```python
from build123d import *

# Parameters (mm, degrees)
F0_W     = 10
F0_H     = 3.175
F0_W_2   = 51.432349664
F0_H_2   = 65
F0_R     = 1.64084
F0_W_3   = 39.0626990616
F0_H_3   = 50
F1_DEPTH = 3.175


# Not quite as in the source:
# - a feature names something its author has since deleted; it is built from what else it names


with BuildPart() as f1:
    # F0 (on Front) → F1 (new body)
    with BuildSketch(Plane.XZ):
        with BuildLine():
            Line((79.2994276966, -35.2024036679), (122.1565705538, -35.2024036679))
            Line((122.1565705538, -35.2024036679), (122.1565705538, 64.7975963321))
            Line((122.1565705538, 64.7975963321), (79.2994276966, 64.7975963321))
            Line((79.2994276966, 64.7975963321), (79.2994276966, 67.9725963321))
            Line((79.2994276966, 67.9725963321), (7.870856268, 67.9725963321))
            Line((7.870856268, 67.9725963321), (7.870856268, 64.7975963321))
            Line((7.870856268, 64.7975963321), (-63.5577151605, 64.7975963321))
            Line((-63.5577151605, 64.7975963321), (-63.5577151605, 67.9725963321))
            Line((-63.5577151605, 67.9725963321), (-134.9862865891, 67.9725963321))
            Line((-134.9862865891, 67.9725963321), (-134.9862865891, 64.7975963321))
            Line((-134.9862865891, 64.7975963321), (-206.4148580177, 64.7975963321))
            Line((-206.4148580177, 64.7975963321), (-206.4148580177, 67.9725963321))
            Line((-206.4148580177, 67.9725963321), (-277.8434294462, 67.9725963321))
            Line((-277.8434294462, 67.9725963321), (-277.8434294462, 64.7975963321))
            Line((-277.8434294462, 64.7975963321), (-277.8434294462, 18.0995963321))
            ThreePointArc((-277.8434294462, 18.0995963321), (-275.5085628548, 17.1324629236), (-274.5414294462, 14.7975963321))
            ThreePointArc((-274.5414294462, 14.7975963321), (-275.5085628548, 12.4627297406), (-277.8434294462, 11.4955963321))
            Line((-277.8434294462, 11.4955963321), (-277.8434294462, -35.2024036679))
            Line((-277.8434294462, -35.2024036679), (-277.8434294462, -38.3774036679))
            Line((-277.8434294462, -38.3774036679), (-206.4148580177, -38.3774036679))
            Line((-206.4148580177, -38.3774036679), (-206.4148580177, -35.2024036679))
            Line((-206.4148580177, -35.2024036679), (-134.9862865891, -35.2024036679))
            Line((-134.9862865891, -35.2024036679), (-134.9862865891, -38.3774036679))
            Line((-134.9862865891, -38.3774036679), (-63.5577151605, -38.3774036679))
            Line((-63.5577151605, -38.3774036679), (-63.5577151605, -35.2024036679))
            Line((-63.5577151605, -35.2024036679), (7.870856268, -35.2024036679))
            Line((7.870856268, -35.2024036679), (7.870856268, -38.3774036679))
            Line((7.870856268, -38.3774036679), (79.2994276966, -38.3774036679))
            Line((79.2994276966, -38.3774036679), (79.2994276966, -35.2024036679))
        make_face()
        with Locations((-247.8332173824, -29.2899036679)):
            Rectangle(F0_W, F0_H, mode=Mode.SUBTRACT)
        with Locations((-227.8332173824, -29.2899036679)):
            Rectangle(F0_W, F0_H, mode=Mode.SUBTRACT)
        with Locations((-239.4272546143, 14.7975963321)):
            Rectangle(F0_W_2, F0_H_2, mode=Mode.SUBTRACT)
        with Locations((63.6818705538, -20.2024036679)):
            Circle(F0_R, mode=Mode.SUBTRACT)
        with Locations((90.6312705538, -20.2024036679)):
            Circle(F0_R, mode=Mode.SUBTRACT)
        Polygon((48.0242208898, -15.8320336679), (48.0242208898, -25.8320336679), (38.0242208898, -25.8320336679), (-193.7110797823, -25.8320336679), (-203.7110797823, -25.8320336679), (-203.7110797823, -15.8320336679), (-203.7110797823, 45.4272263321), (-203.7110797823, 55.4272263321), (-193.7110797823, 55.4272263321), (38.0242208898, 55.4272263321), (48.0242208898, 55.4272263321), (48.0242208898, 45.4272263321), align=None, mode=Mode.SUBTRACT)
        with Locations((77.5555704206, 14.7975963321)):
            Rectangle(F0_W_3, F0_H_3, mode=Mode.SUBTRACT)
        with Locations((-247.8332173824, 58.8850963321)):
            Rectangle(F0_W, F0_H, mode=Mode.SUBTRACT)
        with Locations((-227.8332173824, 58.8850963321)):
            Rectangle(F0_W, F0_H, mode=Mode.SUBTRACT)
        with Locations((63.6818705538, 49.7975963321)):
            Circle(F0_R, mode=Mode.SUBTRACT)
        with Locations((90.6312705538, 49.7975963321)):
            Circle(F0_R, mode=Mode.SUBTRACT)
        Polygon((-203.7110797823, 45.4272263321), (-99.8051057724, 14.7975963321), (-77.8434294462, 21.2715072545), (-193.7110797823, 55.4272263321), (-203.7110797823, 55.4272263321), align=None)
        Polygon((-203.7110797823, -25.8320336679), (-193.7110797823, -25.8320336679), (-77.8434294462, 8.3236854097), (-99.8051057724, 14.7975963321), (-203.7110797823, -15.8320336679), align=None)
        Polygon((38.0242208898, -25.8320336679), (48.0242208898, -25.8320336679), (48.0242208898, -15.8320336679), (-55.8817531201, 14.7975963321), (-77.8434294462, 8.3236854097), align=None)
        Polygon((-55.8817531201, 14.7975963321), (48.0242208898, 45.4272263321), (48.0242208898, 55.4272263321), (38.0242208898, 55.4272263321), (-77.8434294462, 21.2715072545), align=None)
        Polygon((-99.8051057724, 14.7975963321), (-77.8434294462, 8.3236854097), (-55.8817531201, 14.7975963321), (-77.8434294462, 21.2715072545), align=None)
    extrude(amount=F1_DEPTH)


solid = f1.part
```
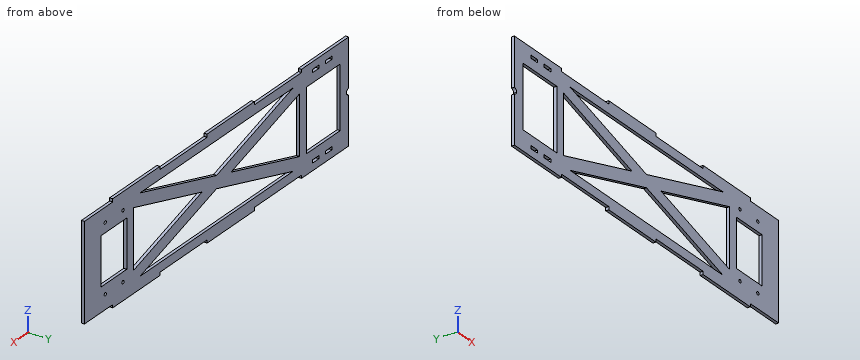
The model under review builds one solid part; all positions refer to its coordinate system, in mm. Round coordinates to 2 decimals unless told otherwise and drop trailing zeros. Loops run counter-clockwise (first coordinate to the right, second up) from the corner with the lowest first, then second, coordinate; pieces in that order, holes last. Notation, with made-up numbers: M 83,35 L 138,35 A38 ccw 138,74 Z; hole C -5.5,63 d6. An arc over 180 degrees is marked long. Write item = value, one per line.
Item 1: Insertion check: P1, Ø1.5, axis at x = -29, y = -2, coming from the +Z side. The pin has a flat end and moves straight along its axis. Give the tip position at first contact, or say it passes through.
Return value:
P1 = 64.8
Item 2: Take a section at C-C on x = -67.5. Write out the cut boundary in (y, z) (3 decimals).
Return value:
outline = M -3.175,-38.377 L 0,-38.377 L 0,-25.832 L -3.175,-25.832 Z; M -3.175,5.275 L 0,5.275 L 0,24.321 L -3.175,24.321 Z; M -3.175,55.427 L 0,55.427 L 0,67.973 L -3.175,67.973 Z
Item 3: Take a section at D-D on x = -183. Write out the cut boundary in (y, z) (3 decimals), then the cut area to 3 significant figures.
Return value:
outline = M -3.175,-35.202 L 0,-35.202 L 0,-25.832 L -3.175,-25.832 Z; M -3.175,-22.675 L 0,-22.675 L 0,-9.727 L -3.175,-9.727 Z; M -3.175,39.322 L 0,39.322 L 0,52.27 L -3.175,52.27 Z; M -3.175,55.427 L 0,55.427 L 0,64.798 L -3.175,64.798 Z
area = 142 mm2
Item 4: For line 1 (Z direction, x = -254, y = -0.8); line 2 (Z direction, x = -15, y = -1.4); line 3 (Z direction, x = 16, y = -2.9), list the stretches that pass through material, from the lowest coordinate up. Write a range as [from, to].
Return value:
line_1 = [-38.38, -17.7], [47.3, 67.97]
line_2 = [-35.2, -25.83], [-10.2, 2.75], [26.85, 39.8], [55.43, 64.8]
line_3 = [-38.38, -25.83], [-19.34, -6.39], [35.99, 48.93], [55.43, 67.97]
Item 5: Take a section at B-B on z = 35.5. Write out the cut boundary in (x, y) (3 decimals).
Return value:
outline = M -277.843,-3.175 L -265.143,-3.175 L -265.143,0 L -277.843,0 Z; M -213.711,-3.175 L -203.711,-3.175 L -203.711,0 L -213.711,0 Z; M -170.035,-3.175 L -126.111,-3.175 L -126.111,0 L -170.035,0 Z; M -29.576,-3.175 L 14.348,-3.175 L 14.348,0 L -29.576,0 Z; M 48.024,-3.175 L 58.024,-3.175 L 58.024,0 L 48.024,0 Z; M 97.087,-3.175 L 122.157,-3.175 L 122.157,0 L 97.087,0 Z
Item 6: Take a section at A-A on x = -239. Write out the cut boundary in (y, z) (3 decimals), then the cut area to 3 significant figures.
Return value:
outline = M -3.175,-38.377 L 0,-38.377 L 0,-17.702 L -3.175,-17.702 Z; M -3.175,47.298 L 0,47.298 L 0,67.973 L -3.175,67.973 Z
area = 131 mm2
